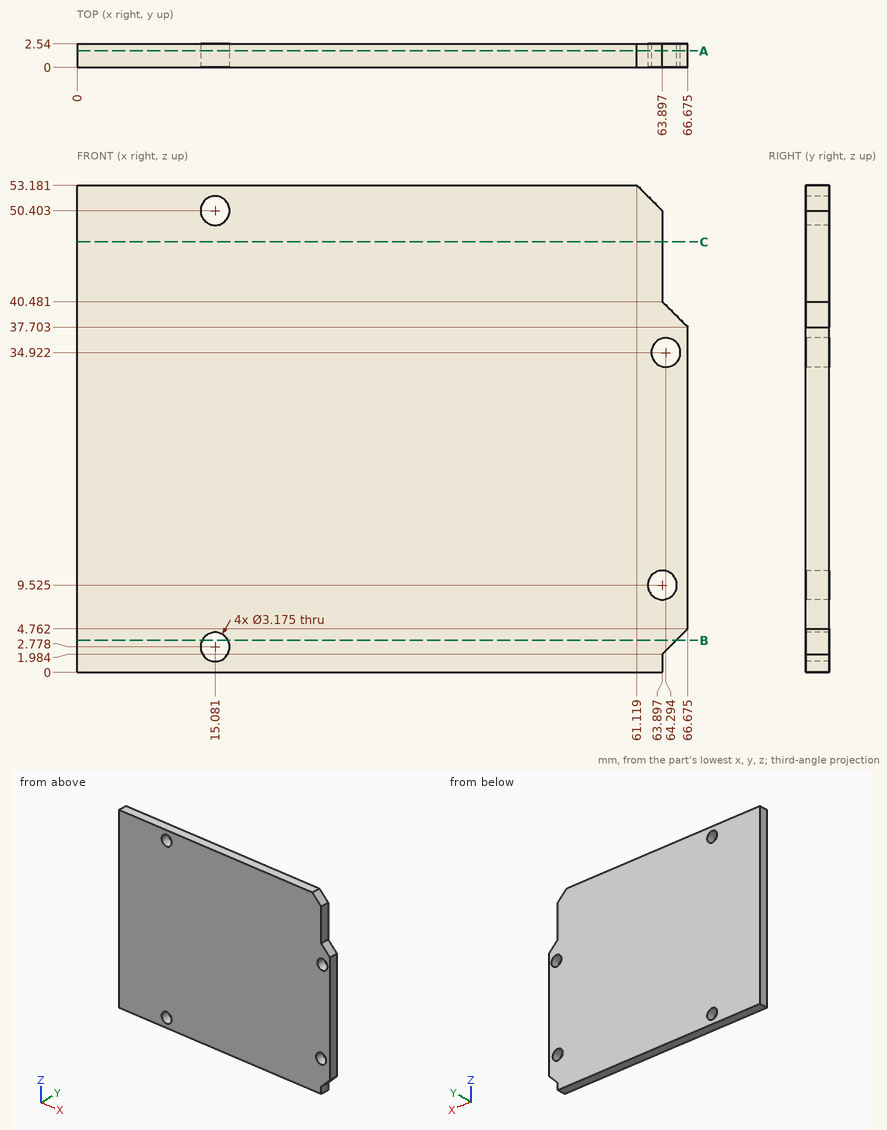
Here's the drawing with two shaded views (mm, measured from the low corner). I have some questions. Round coordinates to 2 decimals unless told otherwise and drop trailing zeros. Write each loop counter-clockwise with the first axis right and the second up, starting at its lowest first coordinate (ties: lowest second). Pieces come first, ordered by that corner, then holes.
(1) Suppose I cut it at C-C on z = 47. Write out the boundary of the cut face in (x, y), and give its area (3 significant figures).
Findings below:
outline: (0, 0) - (63.9, 0) - (63.9, 2.54) - (0, 2.54) - close
area: 162 mm2
(2) Suppose I cut it at B-B on z = 3.5. Write out the boundary of the cut face in (x, y) (1 decimal).
Findings below:
outline: (0, 0) - (13.7, 0) - (13.7, 2.5) - (0, 2.5) - close; (16.5, 0) - (65.4, 0) - (65.4, 2.5) - (16.5, 2.5) - close
(3) For pin 1 (1.9 mm diameter, centred on x = 64.29, z = 34.92, fed in from +Y); pin 2 (0.8 mm diameter, centred on y = 1, z = 44, fed in from +X), each with a flat end and sliding along its axis, tell me the tip position at first contact or that it passes through.
Findings below:
pin 1: passes through
pin 2: stops at x = 63.9
(4) If I drill on probe 1 along X at (y, z) = (2.3, 45.5); probe 2 along X at (y, z) = (1.45, 3) (1 decimal); probe 3 along X at (y, z) = (0.95, 34) (1 decimal), over which ranges is the centre line in solid material (lowest first)?
Findings below:
probe 1: x = 0 to 63.9
probe 2: x = 0 to 13.5, 16.7 to 64.9
probe 3: x = 0 to 63, 65.6 to 66.7
(5) Suppose I cut it at A-A on y = 1.8. Write out the boundary of the cut face in (x, z) (1 decimal).
Findings below:
outline: (0, 0) - (63.9, 0) - (63.9, 2) - (66.7, 4.8) - (66.7, 37.7) - (63.9, 40.5) - (63.9, 50.4) - (61.1, 53.2) - (0, 53.2) - close; hole circle Ø3.2 at (15.1, 2.8); hole circle Ø3.2 at (15.1, 50.4); hole circle Ø3.2 at (63.9, 9.5); hole circle Ø3.2 at (64.3, 34.9)
